The figure shows three views and two pictorial views of one solid part (mm, origin at its lowest corner). Answer the questions. A direction names the side the tool comes from. Coordinates: 2 decimals unless noted, no trailing zeros. Write each loop counter-clockwise with the first axis right and the second up, starting at its lowest first coordinate (ties: lowest second). Pieces come first, ordered by that corner, then holes.
Item 1: Each of these flat-tipped pins is pushed along its axis until it touches: P1, Ø7.5, axis at x = 13.5, y = 15, coming from the +Z side; P2, Ø6, axis at x = 13.5, z = 15, coming from the +Y side; P3, Ø1.5, axis at x = 31.5, y = 12, coming from the -Z side; P4, Ø10, axis at x = 19.5, z = 17, coming from the +Y side. Where does it stop, or does it pass through?
Item 2: Determine the mould class of the marked faces 1, 2 and 3 for opening direction Y: released by +Y, released by -Y, zero draft, split by the parting line, or undercut.
Item 3: Section A-A (x = 13.5) is taken. State how many separate pieces and enclosed holes the cut face has, then the cut area to 3 significant figures.
Item 4: A tool of negligible diameter and unlimited length cuts with its end or side. For the marked faces 4, 5, 6, 7 and 8, from which of +Z, -Z, +X, -X, +Y, -Y can it reach the whole face along a straight path? Write none if from no direction.
Item 5: Straight lines are drawn through the part: probe 1 along X at (y, z) = (15, 1.7) (1 decimal); probe 2 along X at (y, z) = (13.5, 16.25) (1 decimal); probe 3 along Z at (x, y) = (47, 22.5) (1 decimal). For each, find the intervals that lie inside material, in ascending order.
Item 6: Section C-C (x = 31.5) is taken. Give the vertices of the cut face in (y, z).
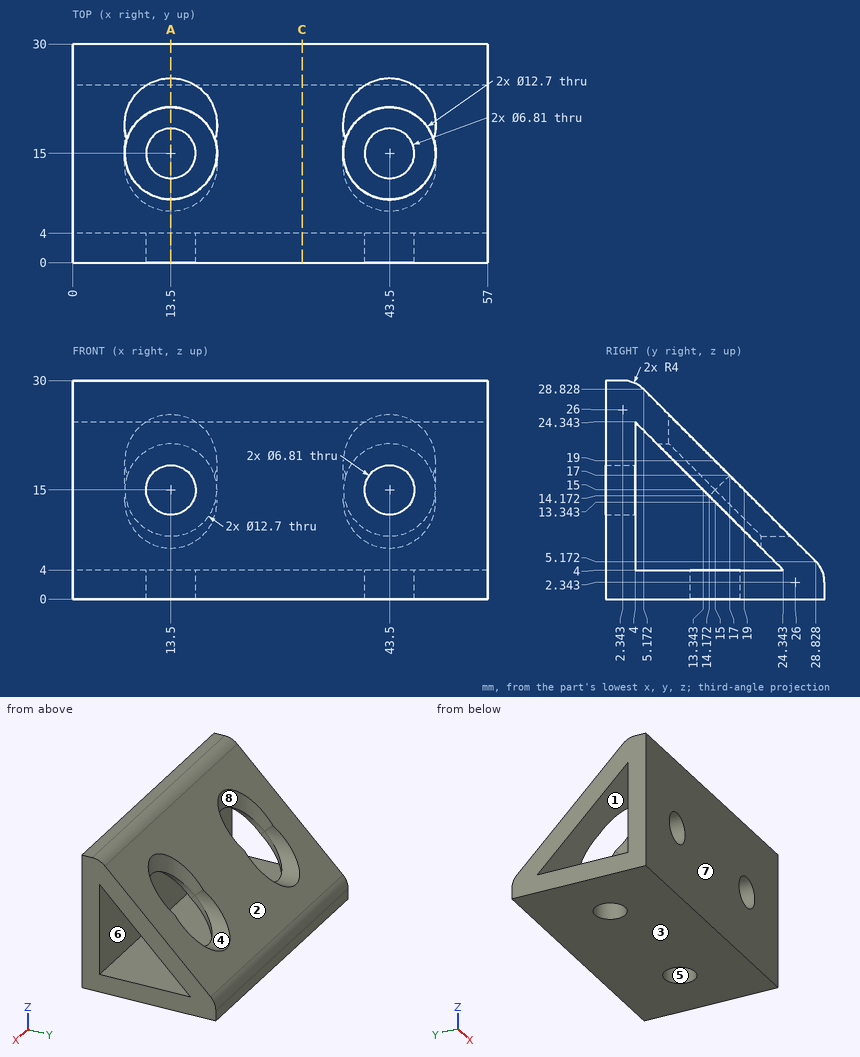
Established:
1. P1: stops at z = 4
1. P2: passes through
1. P3: stops at z = 0
1. P4: stops at y = 22
2. face 1: undercut
2. face 2: released by +Y
2. face 3: zero draft
3. separate pieces: 3
3. enclosed holes: 0
3. area: 219 mm2
4. face 4: +Y
4. face 5: +Z, -Z
4. face 6: +X, -X
4. face 7: +Z, -Z, +X, -X, -Y
4. face 8: +Z
5. probe 1: x = 0 to 10.1, 16.9 to 40.1, 46.9 to 57
5. probe 2: x = 0 to 7.3, 19.7 to 37.3, 49.7 to 57
5. probe 3: z = 0 to 4, 5.8 to 9.7
6. outline: (0, 0) - (30, 0) - (30, 2.34) arc R4 ccw to (28.83, 5.17) - (5.17, 28.83) arc R4 ccw to (2.34, 30) - (0, 30) - close; hole (4, 4) - (24.34, 4) - (4, 24.34) - close
